Autodesk Inventor part; units mm, degrees
ref_plane "YZ Plane" through (0, 0, 0) normal (1, 0, 0) x (0, 1, 0)
ref_plane "XZ Plane" through (0, 0, 0) normal (0, 1, 0) x (-1, 0, 0)
ref_plane "XY Plane" through (0, 0, 0) normal (0, 0, 1) x (1, 0, 0)
sketch "草图1" plane through (0, 0, 0) normal (1, 0, 0) x (0, 1, 0)
  line L0 (35, 150) -> (-35, 150)
  line L1 (-35, 150) -> (-35, -150)
  line L2 (-35, -150) -> (35, -150)
  line L3 (35, -150) -> (35, 150)
  point P0 (0, 0)
  dimension "d0" = 70
  dimension "d1" = 300
extrude "拉伸1" add sketch "草图1" along normal blind 20
sketch "草图2" plane through (0, 35, 150) normal (0, 1, 0) x (1, 0, 0)
  circle A0 centre (10, 50) radius 2
  point P0 (0, 150)
  dimension "d4" = 4
extrude "拉伸2" cut sketch "草图2" against normal blind 20
sketch "草图3" plane through (0, 35, 150) normal (0, 1, 0) x (1, 0, 0)
  circle A0 centre (10, 250) radius 2
  point P0 (0, 150)
  dimension "d7" = 4
extrude "拉伸3" cut sketch "草图3" against normal blind 40
sketch "草图4" plane through (20, 0, 0) normal (1, 0, 0) x (0, 0, -1)
  circle A0 centre (100, 0) radius 3
  point P0 (0, 0)
  dimension "d10" = 6
extrude "拉伸4" cut sketch "草图4" against normal through all
sketch "草图5" plane through (20, 0, 0) normal (1, 0, 0) x (0, 0, -1)
  circle A0 centre (-100, 0) radius 3
  point P0 (0, 0)
  dimension "d13" = 6
extrude "拉伸5" cut sketch "草图5" against normal through all
sketch "草图6" plane through (20, 0, 0) normal (1, 0, 0) x (0, 0, -1)
  circle A0 centre (-100, 0) radius 3
  circle A1 centre (-100, 0) radius 3
  point P0 (0, 0)
  dimension "d16" = 6
extrude "拉伸6" add sketch "草图6" against normal blind 20
sketch "草图7" plane through (20, 0, 0) normal (1, 0, 0) x (0, 0, -1)
  circle A0 centre (100, 0) radius 3
  circle A1 centre (100, 0) radius 3
  point P0 (0, 0)
  dimension "d19" = 6
extrude "拉伸7" add sketch "草图7" against normal blind 20
sketch "草图8" plane through (0, -35, -150) normal (0, -1, 0) x (1, 0, 0)
  line L0 (0, 300) -> (0, 0)
  line L1 (20, 300) -> (20, 0)
  line L2 (0, 300) -> (20, 300)
  line L3 (20, 300) -> (20, 0)
  line L4 (20, 0) -> (0, 0)
  line L5 (0, 0) -> (0, 300)
  point P0 (0, 150)
sketch "草图9" plane through (20, 0, 0) normal (1, 0, 0) x (0, 0, -1)
  circle A0 centre (-100, -15) radius 3
  point P0 (0, 0)
  dimension "d22" = 6
extrude "拉伸8" cut sketch "草图9" against normal through all
sketch "草图10" plane through (20, 0, 0) normal (1, 0, 0) x (0, 0, -1)
  circle A0 centre (100, -15) radius 3
  point P0 (0, 0)
  dimension "d25" = 6
extrude "拉伸9" cut sketch "草图10" against normal through all
sketch "草图11" plane through (20, 0, 0) normal (1, 0, 0) x (0, 0, -1)
  circle A0 centre (-100, -15) radius 3
  circle A1 centre (-100, -15) radius 3
  point P0 (0, 0)
sketch "草图12" plane through (0, -35, -150) normal (0, -1, 0) x (1, 0, 0)
  point P0 (0, 150)
sketch "草图13" plane through (0, -35, -150) normal (0, -1, 0) x (1, 0, 0)
  point P0 (0, 150)
properties part number "马达安装版"
Build history of the part. All positions in model axes, mm. Coordinates: 2 decimals unless noted, no trailing zeros. Order: outer loops, then holes, each group sorted by start corner. A loop starts at its lowest first (then second) coordinate and runs counter-clockwise, first axis right, second up. Notation, with made-up numbers: (29.5, 37.5) - (75.5, 37.5) arc R25 ccw to (75.5, 57.5) - close; hole circle Ø8 at (10, 3.5). An arc over 180 degrees is marked (long way). Write each question's results on one line, items separated by ' | '. Start each with the question number.
Item 1: Flat gauge pins, fed straight in: pin 1 (3 mm diameter, centred on x = 10, z = -100, fed in from +Y); pin 2 (1.2 mm diameter, centred on x = 10.5, z = 100, fed in from +Y). Where does each tip first touch, or does it go through?
Item 2: Band-saw the part on A-A on y = -15. Write the cut outline in (x, z).
Item 3: Mould opens along Z. For faces 1 (the face through (10.1, -16.8, 102.4)), 2 (the face through (10, 0, 150)), 3 (the face through (10, -35, 2)), 4 (the face through (10, 0, -150)) say: released by +Z, released by -Z, zero draft, split by the parting line, or undercut.
Item 4: Wall check: probe 1 along Z at (x, y) = (6, -14.5); probe 2 along Z at (x, y) = (10, 24.5); probe 3 along Z at (x, y) = (10, 11). Give the ranges that are in metal, low to high. Write a range as [from, to].
Numbers:
1) pin 1: y = 3 | pin 2: y = 15
2) outline: (0, -150) - (20, -150) - (20, -103) - (0, -103) - close; (0, -97) - (20, -97) - (20, 97) - (0, 97) - close; (0, 103) - (20, 103) - (20, 150) - (0, 150) - close
3) face 1: undercut | face 2: released by +Z | face 3: zero draft | face 4: released by -Z
4) probe 1: [-150, -102.96], [-97.04, 97.04], [102.96, 150] | probe 2: [-150, -102], [-98, 98], [102, 150] | probe 3: [-150, -102], [-98, 150]
